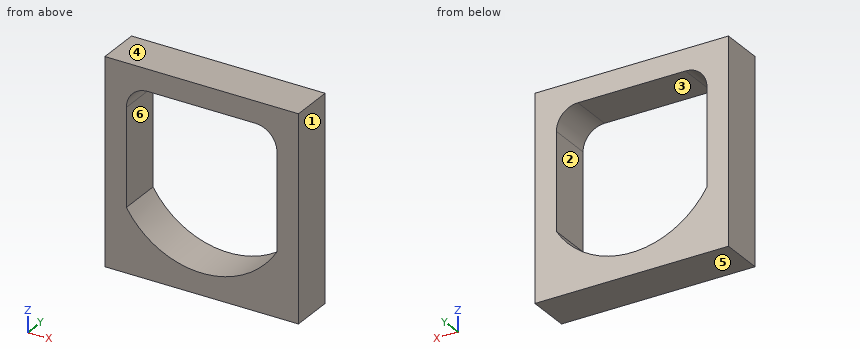
```python
from build123d import *

# Parameters (mm, degrees)
F0_W     = 90
F0_H     = 94.526901
F1_DEPTH = 20


with BuildPart() as f1:
    # F0 (on Front) → F1 (new body)
    with BuildSketch(Plane.XZ):
        with Locations((10.317164, -11.026002)):
            Rectangle(F0_W, F0_H)
        with BuildLine():
            ThreePointArc((-24.682836, 16.237448), (-21.753904, 23.308516), (-14.682836, 26.237448))
            Line((-14.682836, 26.237448), (35.317164, 26.237448))
            ThreePointArc((35.317164, 26.237448), (42.388231, 23.308516), (45.317164, 16.237448))
            Line((45.317164, 16.237448), (45.317164, -28.762552))
            ThreePointArc((45.317164, -28.762552), (10.317164, -48.289453), (-24.682836, -28.762552))
            Line((-24.682836, -28.762552), (-24.682836, 16.237448))
        make_face(mode=Mode.SUBTRACT)
    extrude(amount=F1_DEPTH)


solid = f1.part
```
For this review, take the finished solid that the model builds, in its own axes (mm). Face numbers are marked on the shaded views. A direction names the side the tool comes from. Give positions to 0.01 mm unless a question says otherwise; leave off trailing zeros. Order: outer loops, then holes, each group sorted by start corner. A loop starts at its lowest first (then second) coordinate and runs counter-clockwise, first axis right, second up.
1) Take a section at B-B (x = 9.5). Give the boundary of the cut face in (y, z).
2) The part is to be moulded in two halves that separate along Z. For the marked faces 1, 2, 3 and 4, say which applies: released by +Z, released by -Z, zero draft, split by the parting line, or undercut.
3) Take a section at A-A (z = -9.5). Give the boundary of the cut face in (x, y), then the cut area to 3 significant figures.
4) For the marked faces 5 and 6, list the 3-axis set-ups (+Z, -Z, +X, -X, +Y, -Y) from which the entire face can be reached by the end or side of a thin tool; tool diameter is ignored.
5) Wall thickness on line 1 (Z direction, x = 9, y = -8.5); line 2 (X direction, y = -17.25, z = -5.5); line 3 (Z direction, x = -2.5, y = -5.75): over which ranges is each line inside the solid? List them lowest first.
6) Take a section at C-C (y = -7.5). Give the boundary of the cut face in (x, z).
Derived:
1. outline: (-20, -58.29) - (0, -58.29) - (0, -48.28) - (-20, -48.28) - close; (-20, 26.24) - (0, 26.24) - (0, 36.24) - (-20, 36.24) - close
2. face 1: zero draft
2. face 2: undercut
2. face 3: undercut
2. face 4: released by +Z
3. outline: (-34.68, -20) - (-24.68, -20) - (-24.68, 0) - (-34.68, 0) - close; (45.32, -20) - (55.32, -20) - (55.32, 0) - (45.32, 0) - close
3. area: 400 mm2
4. face 5: -Z, +X, -X, +Y, -Y
4. face 6: +Y, -Y
5. line 1: z = -58.29 to -48.27, 26.24 to 36.24
5. line 2: x = -34.68 to -24.68, 45.32 to 55.32
5. line 3: z = -58.29 to -46.24, 26.24 to 36.24
6. outline: (-34.68, -58.29) - (55.32, -58.29) - (55.32, 36.24) - (-34.68, 36.24) - close; hole (-24.68, -28.76) arc R41.13 ccw to (45.32, -28.76) - (45.32, 16.24) arc R10 ccw to (35.32, 26.24) - (-14.68, 26.24) arc R10 ccw to (-24.68, 16.24) - close
